Print and shaded views of the part. All mm, measured from the part's lowest x, y and z. A direction names the side the tool comes from. Give positions to 0.01 mm unless a question says otherwise; leave off trailing zeros. Loops run counter-clockwise (first coordinate to the right, second up) from the corner with the lowest first, then second, coordinate; pieces in that order, holes last. Notation, with made-up numbers: (79, 74.5) - (130, 74.5) arc R9 cw to (130, 90.5) - close; hole circle Ø3 at (-1.75, -35.5). An arc over 180 degrees is marked (long way). Return JSON: item names as keys, results as strings.
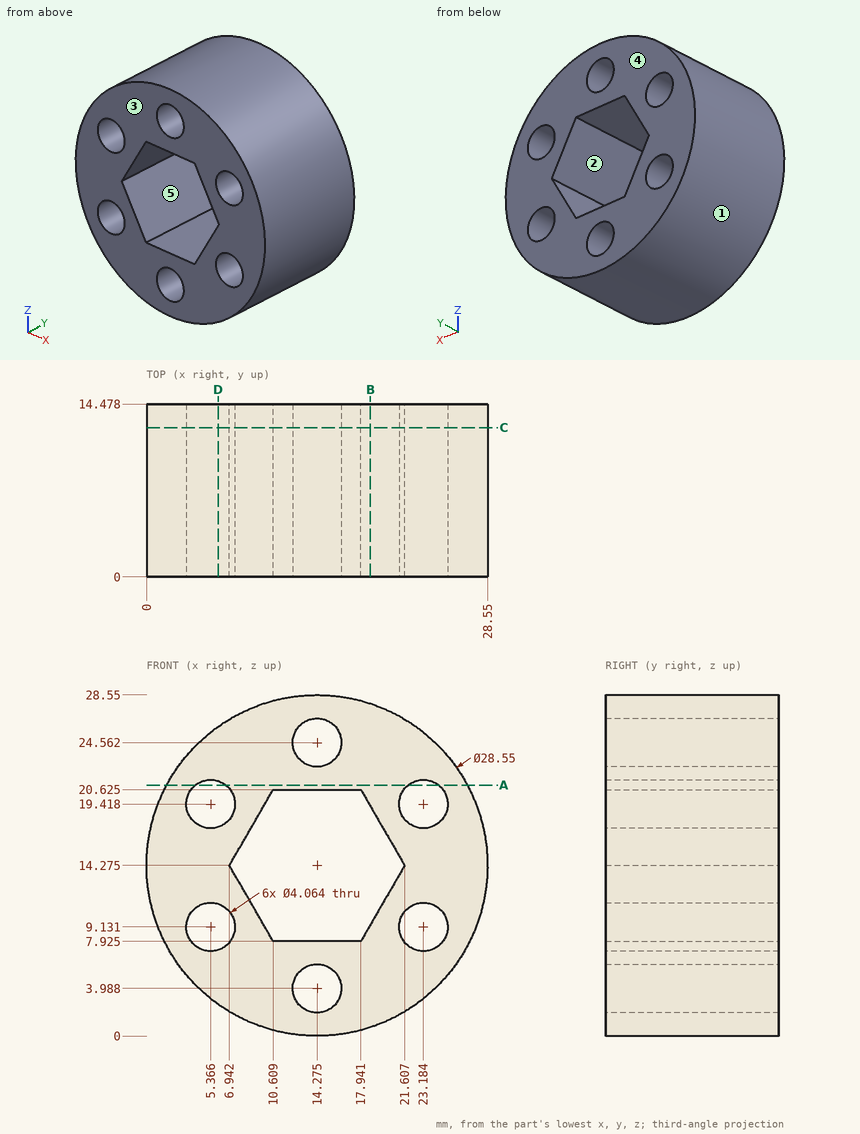
1. Cut at B-B, the plane x = 18.75. Write the cut outline in (y, z), plus the area to 3 significant figures.
Values follow:
{"outline": "(0, 0.72) - (14.48, 0.72) - (14.48, 9.33) - (0, 9.33) - close; (0, 19.22) - (14.48, 19.22) - (14.48, 27.83) - (0, 27.83) - close", "area": "249 mm²"}
2. Cut at C-C, the plane y = 12.5. Give the number of separate pieces and of enclosed holes in the cut face.
Values follow:
{"separate pieces": "1", "enclosed holes": "7"}
3. Cut at A-A, the plane z = 21. Write the cut outline in (x, y), plus the area to 3 significant figures.
Values follow:
{"outline": "(1.68, 0) - (4.09, 0) - (4.09, 14.48) - (1.68, 14.48) - close; (6.64, 0) - (21.91, 0) - (21.91, 14.48) - (6.64, 14.48) - close; (24.46, 0) - (26.87, 0) - (26.87, 14.48) - (24.46, 14.48) - close", "area": "291 mm²"}
4. Drill centre lines: probe 1 along X at (y, z) = (2.25, 19.5) (1 decimal); probe 2 along Z at (x, y) = (5.25, 11.25) (1 decimal); probe 3 along Z at (x, y) = (4, 12.75) (1 decimal). Where is each one in solid material? Low to high.
Values follow:
{"probe 1": "x = 1 to 3.3, 7.4 to 10, 18.6 to 21.2, 25.2 to 27.6", "probe 2": "z = 3.2 to 7.1, 11.2 to 17.4, 21.4 to 25.3", "probe 3": "z = 4.4 to 7.6, 10.6 to 17.9, 20.9 to 24.2"}
5. Cut at D-D, the plane x = 6. Write the cut outline in (y, z), plus the area to 3 significant figures.
Values follow:
{"outline": "(0, 2.64) - (14.48, 2.64) - (14.48, 7.2) - (0, 7.2) - close; (0, 11.06) - (14.48, 11.06) - (14.48, 17.49) - (0, 17.49) - close; (0, 21.35) - (14.48, 21.35) - (14.48, 25.91) - (0, 25.91) - close", "area": "225 mm²"}
6. Which spindle directions (+Z, -Z, +X, -X, +Y, -Y) get a long thin tool onto all of the face, cutting with end or side? Do the marked faces 4 and 5. Say none if no direction does.
Values follow:
{"face 4": "+Z, -Z, +X, -X, +Y", "face 5": "+Y, -Y"}
7. Pull direction X, two halves, no side cores. Call the marked faces 1, 2 and 3: +X half, -X half, draft (parallel to the pull), parting line (faces both ways), or undercut.
Values follow:
{"face 1": "parting line", "face 2": "undercut", "face 3": "draft"}
8. Drop flat-ended pins along their axis: P1, Ø2.5, axis at x = 5.37, z = 19.42, coming from the +Y side; P2, Ø6, axis at x = 23.5, y = 7, coming from the -Z side; P3, Ø1, axis at x = 12.5, y = 8.5, coming from the +Z side; P4, Ø1, axis at y = 3.5, z = 16, coming from the -X side. Give the stop position or say it passes through.
Values follow:
{"P1": "passes through", "P2": "stops at z = 1.43", "P3": "stops at z = 28.49", "P4": "stops at x = 0.05"}
